For this review, take the finished solid that the model builds, in its own axes (mm). Face numbers are marked on the shaded views. A direction names the side the tool comes from. Coordinates: 2 decimals unless noted, no trailing zeros. Write each loop counter-clockwise with the first axis right and the second up, starting at its lowest first coordinate (ties: lowest second). Pieces come first, ordered by that corner, then holes. Notation, with made-up numbers: (-26, -0.5) - (-7, -0.5) arc R14 cw to (-7, 6.5) - close; hole circle Ø5 at (68, 82.25). An arc over 180 degrees is marked (long way). Write each question's results on one line, items separated by ' | '.
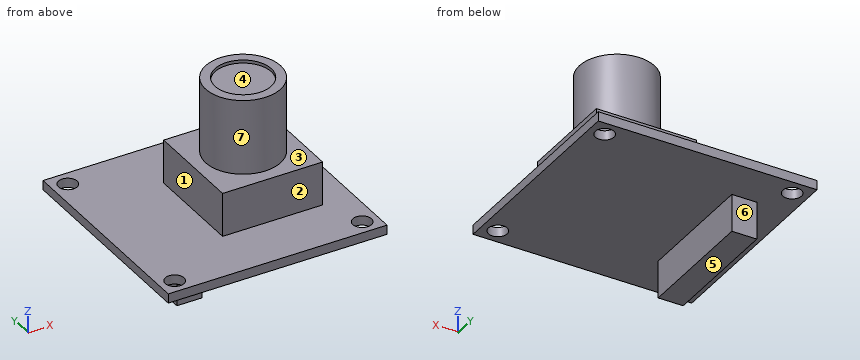
from build123d import *

# Parameters (mm, degrees)
SKETCH1_W           = 35
SKETCH1_H           = 34
BOSS_EXTRUDE1_DEPTH = 1.5
CUT_EXTRUDE1_REACH  = 3.5
SKETCH2_R           = 1.5
SKETCH3_W           = 16
SKETCH3_H           = 16
BOSS_EXTRUDE3_DEPTH = 7
SKETCH4_R           = 6
BOSS_EXTRUDE4_DEPTH = 12
SKETCH7_R           = 4.5
CUT_EXTRUDE2_DEPTH  = 0.5
SKETCH8_W           = 4
SKETCH8_H           = 20
BOSS_EXTRUDE5_DEPTH = 6


with BuildPart() as part:
    # Sketch1 → Boss-Extrude1 (new body)
    with BuildSketch(Plane.XY):
        Rectangle(SKETCH1_W, SKETCH1_H)
    extrude(amount=-BOSS_EXTRUDE1_DEPTH)

    # Sketch2 → Cut-Extrude1 (cut, up to next)
    with BuildSketch(Plane.XY, mode=Mode.PRIVATE) as cut_extrude1_sk1:
        with Locations((-15, -14.5)):
            Circle(SKETCH2_R)
    cut_extrude1_tool1 = extrude(cut_extrude1_sk1.sketch, amount=-CUT_EXTRUDE1_REACH, mode=Mode.PRIVATE) & part.part
    add(cut_extrude1_tool1.solids().sort_by_distance((-15, -14.5, 0))[0], mode=Mode.SUBTRACT)
    # Sketch2 → Cut-Extrude1 (cut, up to next)
    with BuildSketch(Plane.XY, mode=Mode.PRIVATE) as cut_extrude1_sk2:
        with Locations((15, -14.5)):
            Circle(SKETCH2_R)
    cut_extrude1_tool2 = extrude(cut_extrude1_sk2.sketch, amount=-CUT_EXTRUDE1_REACH, mode=Mode.PRIVATE) & part.part
    add(cut_extrude1_tool2.solids().sort_by_distance((15, -14.5, 0))[0], mode=Mode.SUBTRACT)
    # Sketch2 → Cut-Extrude1 (cut, up to next)
    with BuildSketch(Plane.XY, mode=Mode.PRIVATE) as cut_extrude1_sk3:
        with Locations((15, 14.5)):
            Circle(SKETCH2_R)
    cut_extrude1_tool3 = extrude(cut_extrude1_sk3.sketch, amount=-CUT_EXTRUDE1_REACH, mode=Mode.PRIVATE) & part.part
    add(cut_extrude1_tool3.solids().sort_by_distance((15, 14.5, 0))[0], mode=Mode.SUBTRACT)
    # Sketch2 → Cut-Extrude1 (cut, up to next)
    with BuildSketch(Plane.XY, mode=Mode.PRIVATE) as cut_extrude1_sk4:
        with Locations((-15, 14.5)):
            Circle(SKETCH2_R)
    cut_extrude1_tool4 = extrude(cut_extrude1_sk4.sketch, amount=-CUT_EXTRUDE1_REACH, mode=Mode.PRIVATE) & part.part
    add(cut_extrude1_tool4.solids().sort_by_distance((-15, 14.5, 0))[0], mode=Mode.SUBTRACT)

    # Sketch3 → Boss-Extrude3 (add)
    with BuildSketch(Plane.XY):
        with Locations((4.5, 0)):
            Rectangle(SKETCH3_W, SKETCH3_H)
    extrude(amount=BOSS_EXTRUDE3_DEPTH)

    # Sketch4 → Boss-Extrude4 (add)
    with BuildSketch(Plane.XY.offset(7)):
        with Locations((4.5, 0)):
            Circle(SKETCH4_R)
    extrude(amount=BOSS_EXTRUDE4_DEPTH)

    # Sketch7 → Cut-Extrude2 (cut)
    with BuildSketch(Plane.XY.offset(19)):
        with Locations((4.5, 0)):
            Circle(SKETCH7_R)
    extrude(amount=-CUT_EXTRUDE2_DEPTH, mode=Mode.SUBTRACT)

    # Sketch8 → Boss-Extrude5 (add)
    with BuildSketch(Plane(origin=(0, 0, -1.5), x_dir=(-1, 0, 0), z_dir=(0, 0, -1))):
        with Locations((10, 0)):
            Rectangle(SKETCH8_W, SKETCH8_H)
    extrude(amount=BOSS_EXTRUDE5_DEPTH)


solid = part.part
Q1. Wall thickness on line 1 along Y through (x, z) = (15, -0.55); line 2 along Y through (x, z) = (4.5, 18.95); line 3 along Z through (x, y) = (-2, -5.5): over which ranges is each line inside the solid? List them lowest first. Write a range as from..to.
Results found:
line 1: -17..-16, -13..13, 16..17 | line 2: -6..-4.5, 4.5..6 | line 3: -1.5..7
Q2. Take a section at B-B on x = -15. State the section outline as (y, z) points, plus the area to 3 significant figures.
Results found:
outline: (-17, -1.5) - (-16, -1.5) - (-16, 0) - (-17, 0) - close; (-13, -1.5) - (13, -1.5) - (13, 0) - (-13, 0) - close; (16, -1.5) - (17, -1.5) - (17, 0) - (16, 0) - close | area: 42.0 mm2
Q3. For pin 1 (8 mm diameter, centred on x = 4.5, y = 0, fed in from -Z); pin 2 (7 mm diameter, centred on x = 2.5, y = -1, fed in from +Z); pin 3 (2 mm diameter, centred on x = -10, z = -5, fed in from +Y); pin 4 (5.5 mm diameter, centred on y = -0.5, z = 3, fed in from +X), all flat-tipped, find the tip position at first contact; note any pin that passes through.
Results found:
pin 1: z = -1.5 | pin 2: z = 19 | pin 3: y = 10 | pin 4: x = 12.5
Q4. Take a section at A-A on y = -14.5. State the section outline as (x, z) points, plus the area to 3 significant figures.
Results found:
outline: (-17.5, -1.5) - (-16.5, -1.5) - (-16.5, 0) - (-17.5, 0) - close; (-13.5, -1.5) - (13.5, -1.5) - (13.5, 0) - (-13.5, 0) - close; (16.5, -1.5) - (17.5, -1.5) - (17.5, 0) - (16.5, 0) - close | area: 43.5 mm2
Q5. Take a section at D-D on y = 0. State the section outline as (x, z) points.
Results found:
outline: (-17.5, -1.5) - (-12, -1.5) - (-12, -7.5) - (-8, -7.5) - (-8, -1.5) - (17.5, -1.5) - (17.5, 0) - (12.5, 0) - (12.5, 7) - (10.5, 7) - (10.5, 19) - (9, 19) - (9, 18.5) - (0, 18.5) - (0, 19) - (-1.5, 19) - (-1.5, 7) - (-3.5, 7) - (-3.5, 0) - (-17.5, 0) - close
Q6. Take a section at C-C on x = -3. State the section outline as (y, z) points.
Results found:
outline: (-17, -1.5) - (17, -1.5) - (17, 0) - (8, 0) - (8, 7) - (-8, 7) - (-8, 0) - (-17, 0) - close
Q7. For the marked faces 1, 2 and 3, list the 3-axis set-ups (+Z, -Z, +X, -X, +Y, -Y) from which the entire face can be reached by the end or side of a thin tool; tool diameter is ignored.
Results found:
face 1: +Z, -X, +Y, -Y | face 2: +Z, +X, -X, -Y | face 3: +Z
Q8. Mouldability with a two-part tool opening along Y and no side actions: class the marked faces 4, 5, 6 and 7 as pulls with the +Y half, pulls with the -Y half, needs draft (parallel to the pull), parting line crosses it, or undercut.
Results found:
face 4: undercut | face 5: needs draft | face 6: pulls with the +Y half | face 7: parting line crosses it
